The drawing under review shows one solid part. Ordinate dimensions are in mm from its lowest x, y, z. Coordinates: 2 decimals unless noted, no trailing zeros. Write each loop counter-clockwise with the first axis right and the second up, starting at its lowest first coordinate (ties: lowest second). Pieces come first, ordered by that corner, then holes.
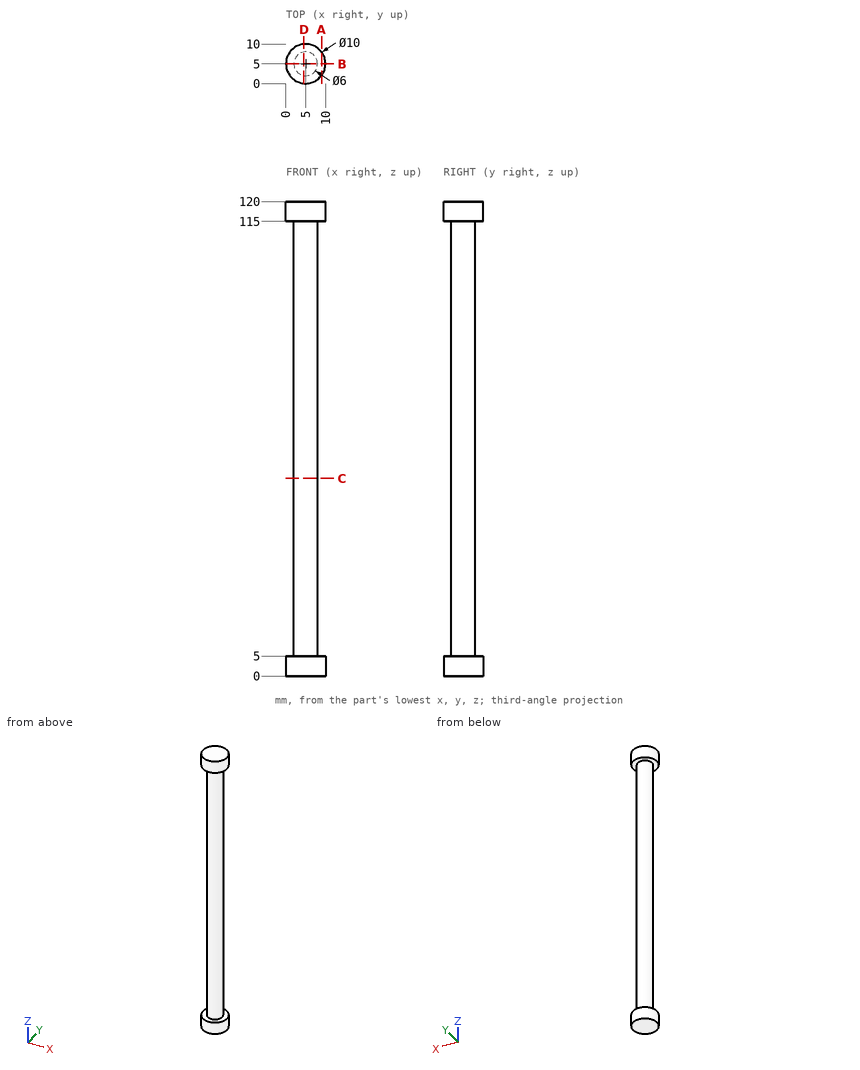
Q1. Add section A-A (x = 9). State the section outline as (y, z) points, then the cut area to 3 significant figures.
Ans:
outline: (2, 0) - (8, 0) - (8, 5) - (2, 5) - close; (2, 115) - (8, 115) - (8, 120) - (2, 120) - close
area: 60.0 mm2
Q2. Add section C-C (z = 50). State the section outline as (x, y) points.
Ans:
outline: circle Ø6 at (5, 5)
Q3. Add section B-B (y = 5). State the section outline as (x, z) points, then the cut area to 3 significant figures.
Ans:
outline: (0, 0) - (10, 0) - (10, 5) - (8, 5) - (8, 115) - (10, 115) - (10, 120) - (0, 120) - (0, 115) - (2, 115) - (2, 5) - (0, 5) - close
area: 760 mm2
Q4. Clearance check with flat-ended pins moving along their axes: pin 1 Ø3 at (x, y) = (6, 7.5) entering from -Z; pin 2 Ø2 at (y, z) = (5, 77.5) entering from +X; pin 3 Ø6 at (x, z) = (2, 95.5) entering from -Y; pin 4 Ø5 at (y, z) = (4, 29.5) entering from -X. State where each tip first meets the part, or that it passes through.
Ans:
pin 1: stops at z = 0
pin 2: stops at x = 8
pin 3: stops at y = 2
pin 4: stops at x = 2
Q5. For probe 1 along Z at (x, y) = (4.5, 1.5); probe 2 along Y at (x, z) = (7, 22.5); probe 3 along Y at (x, z) = (6, 26), list the stretches that pass through material, from the lowest coordinate up.
Ans:
probe 1: z = 0 to 5, 115 to 120
probe 2: y = 2.76 to 7.24
probe 3: y = 2.17 to 7.83
Q6. Add section D-D (x = 4.5). State the section outline as (y, z) points.
Ans:
outline: (0.03, 0) - (9.97, 0) - (9.97, 5) - (7.96, 5) - (7.96, 115) - (9.97, 115) - (9.97, 120) - (0.03, 120) - (0.03, 115) - (2.04, 115) - (2.04, 5) - (0.03, 5) - close
